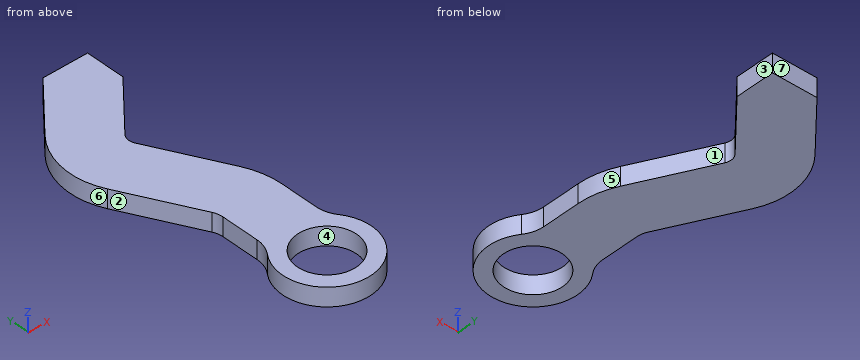
Autodesk Inventor part; units mm, degrees
ref_plane "YZ Plane" through (0, 0, 0) normal (1, 0, 0) x (0, 1, 0)
ref_plane "XZ Plane" through (0, 0, 0) normal (0, 1, 0) x (-1, 0, 0)
ref_plane "XY Plane" through (0, 0, 0) normal (0, 0, 1) x (1, 0, 0)
sketch "Sketch1" plane through (0, 0, 0) normal (0, 0, 1) x (1, 0, 0)
  line L0 (0, 0) -> (2.8584, 0)
  line L1 (0, 0) -> (0, 3.8884)
  circle A0 centre (0, -12.5) radius 4
  arc A1 (-4.8, -8.9) -> (4.8, -8.9) centre (0, -12.5) ccw
  line L2 (4, -1.4002) -> (4, -6.5)
  line L3 (-9.4657, 9.7101) -> (-4.3072, -0.1501)
  arc A2 (-4, -1.4002) -> (-4.3072, -0.1501) centre (-6.6968, -1.4002) ccw
  line L4 (-4, -1.4002) -> (-4, -6.5)
  line L5 (4, -6.5) -> (4, -1.4002)
  arc A3 (4, -1.4002) -> (2.7813, 3.5584) centre (-6.6968, -1.4002) ccw
  line L6 (2.7813, 3.5584) -> (-2.3771, 13.4186)
  arc A4 (-2.17, 15.1733) -> (-2.3771, 13.4186) centre (-0.9897, 14.1444) ccw
  line L7 (-2.17, 15.1733) -> (4, 22.2516)
  line L8 (4, 22.2516) -> (4, 27.5083)
  line L9 (4, 27.5083) -> (-2.0305, 27.5083)
  line L10 (-2.0305, 27.5083) -> (-8.2005, 20.4299)
  arc A5 (-8.2005, 20.4299) -> (-9.4657, 9.7101) centre (-0.9897, 14.1444) ccw
  line L11 (-4, -6.5) -> (-4, -1.4002)
  arc A6 (-4.8, -8.9) -> (-4, -6.5) centre (-8, -6.5) ccw
  arc A7 (4, -6.5) -> (4.8, -8.9) centre (8, -6.5) ccw
  dimension "d1" = 8
  dimension "d16" = 8
  dimension "d17" = 8
  dimension "d18" = 25
  dimension "d19" = 4
  dimension "d20" = 2
  dimension "d21" = 2.8003
  dimension "d22" = 13.3936
  dimension "d23" = 1.9794
  dimension "d24" = 28.2888
  dimension "d25" = 0
extrude "Extrusion1" add sketch "Sketch1" along normal blind 2.5
properties part number "gripper" material "Polystyrene"
Check sheet for the modelled part. Datum: model origin and axes. Units: mm. Face numbers are marked on the shaded views. A direction names the side the tool comes from. Coordinates: 2 decimals unless noted, no trailing zeros. Order: outer loops, then holes, each group sorted by start corner. A loop starts at its lowest first (then second) coordinate and runs counter-clockwise, first axis right, second up. Notation, with made-up numbers: (40.25, 30.5) -> (97.25, 30.5) arc R17 ccw to (97.25, 52.5) -> close; hole circle Ø1 at (47.5, -37.75). An arc over 180 degrees is marked (long way). Write item = value, one per line. Start each with the question number.
1) Material ranges on L1, parallel to Y at x = 0, z = 0.75; L2, parallel to Y at x = 1.25, z = 1.8; L3, parallel to Y at x = -5.5, z = 2.45, recorded low to high.
2) Cross-section at D-D (x = 2). Enter the section's corners in (y, z).
3) Cross-section at A-A (y = -12.5). Enter the section's corners in (x, z), then the cut area to 3 significant figures.
4) Access from +Z, -Z, +X, -X, +Y, -Y to the whole of each face (thin tool, end or side, straight path). Record for the marked faces 1, 2 and 3.
5) Cross-section at C-C (z = 1.25). Enter the section's corners in (x, y), then the cut area to 3 significant figures.
6) Mould release check, pull along X, two halves, no side actions. Record for the marked faces 4, 5, 6 and 7: +X half, -X half, draft (parallel to the pull), parting line (faces both ways), or undercut.
7) Go/stop test with flat-tipped pins: P1, Ø1, axis at y = -12.5, z = 1.5, coming from the -X side; P2, Ø1.2, axis at y = -3, z = 1, coming from the +X side; P3, Ø1.2, axis at y = -3.5, z = 1, coming from the -X side. Record where each tip stops, or that it passes through.
8) Cross-section at B-B (x = 0). Enter the section's corners in (y, z), then the cut area to 3 significant figures.
Ans:
q1.L1 = -18.5 to -16.5, -8.5 to 8.87, 17.66 to 27.51
q1.L2 = -18.37 to -16.3, -8.7 to 6.49, 19.1 to 27.51
q1.L3 = -14.9 to -10.1, 2.13 to 23.53
q2.outline = (-18.16, 0) -> (-15.96, 0) -> (-15.96, 2.5) -> (-18.16, 2.5) -> close; (-9.04, 0) -> (5.05, 0) -> (5.05, 2.5) -> (-9.04, 2.5) -> close; (19.96, 0) -> (27.51, 0) -> (27.51, 2.5) -> (19.96, 2.5) -> close
q3.outline = (-6, 0) -> (-4, 0) -> (-4, 2.5) -> (-6, 2.5) -> close; (4, 0) -> (6, 0) -> (6, 2.5) -> (4, 2.5) -> close
q3.area = 10.0 mm²
q4.face_1 = +Z, -Z, +X
q4.face_2 = +Z, -Z, -X
q4.face_3 = +Z, -Z, +X, +Y
q5.outline = (-9.47, 9.71) -> (-4.31, -0.15) arc R2.7 cw to (-4, -1.4) -> (-4, -6.5) arc R4 cw to (-4.8, -8.9) arc R6 ccw (long way) to (4.8, -8.9) arc R4 cw to (4, -6.5) -> (4, -1.4) arc R10.7 ccw to (2.78, 3.56) -> (-2.38, 13.42) arc R1.57 cw to (-2.17, 15.17) -> (4, 22.25) -> (4, 27.51) -> (-2.03, 27.51) -> (-8.2, 20.43) arc R9.57 ccw to start; hole circle Ø8 at (0, -12.5)
q5.area = 367 mm²
q6.face_4 = undercut
q6.face_5 = +X half
q6.face_6 = -X half
q6.face_7 = draft
q7.P1 = -6
q7.P2 = 4
q7.P3 = -4
q8.outline = (-18.5, 0) -> (-16.5, 0) -> (-16.5, 2.5) -> (-18.5, 2.5) -> close; (-8.5, 0) -> (8.87, 0) -> (8.87, 2.5) -> (-8.5, 2.5) -> close; (17.66, 0) -> (27.51, 0) -> (27.51, 2.5) -> (17.66, 2.5) -> close
q8.area = 73.1 mm²
